The listing builds one solid part. Answer for the finished solid, in the listing's coordinates (mm). Coordinates: 2 decimals unless noted, no trailing zeros. Write each loop counter-clockwise with the first axis right and the second up, starting at its lowest first coordinate (ties: lowest second). Pieces come first, ordered by that corner, then holes.
(1) The part is cut by section B-B on x = 23. Determine the outline of the cut face in (y, z).
(2) The part is cut by section A-A on x = -36. Determine the outline of the cut face in (y, z), plus the area to 3 significant figures.
(3) Straight lines are drawn through the part: line 1 (X direction, y = -26.5, z = 0.5); line 2 (Y direction, x = 54, z = 0.8); line 3 (Y direction, x = 51.5, z = 2.55). For each, find the intervals that lie inside material, in ascending order.
(4) Given P1, Ø1.2, axis at y = 30, z = 3, coming from the -X side; P2, Ø2, axis at x = 57.5, z = 2.5, coming from the -Y side; P3, Ø2, axis at y = -22, z = 0.5, coming from the +X side, each flat-ended and moving along its own axis, determine where each tip first touches the part or whether it passes through.
(5) The part is cut by section C-C on z = 3.1. Give the number of separate pieces and of enclosed holes in the cut face, plus the area to 3 significant figures.
from build123d import *

# Parameters (mm, degrees)
EXTRUDE_1_DEPTH     = 4
CUT_EXTRUDE_1_DEPTH = 10


with BuildPart() as part:
    # 草图1 → 凸台-拉伸1 (new body)
    with BuildSketch(Plane.XY):
        Polygon((55.534285714, 24.23), (59.534285714, 24.23), (59.534285714, 16.23), (55.534285714, 16.23), (55.534285714, 6.73), (51.534285714, 6.73), (51.534285714, 8.08), (48.934285714, 8.08), (48.934285714, 6.73), (46.934285714, 6.73), (46.934285714, 3.73), (48.934285714, 3.73), (48.934285714, 2.38), (51.534285714, 2.38), (51.534285714, 3.73), (55.534285714, 3.73), (55.534285714, -5.77), (59.534285714, -5.77), (59.534285714, -13.77), (55.534285714, -13.77), (55.534285714, -23.27), (51.534285714, -23.27), (51.534285714, -21.92), (48.934285714, -21.92), (48.934285714, -23.27), (46.934285714, -23.27), (46.934285714, -26.27), (48.934285714, -26.27), (48.934285714, -27.62), (51.534285714, -27.62), (51.534285714, -26.27), (55.534285714, -26.27), (55.534285714, -35.77), (-70.465714286, -35.77), (-70.465714286, -26.27), (-66.465714286, -26.27), (-66.465714286, -27.62), (-63.865714286, -27.62), (-63.865714286, -26.27), (-61.865714286, -26.27), (-61.865714286, -23.27), (-63.865714286, -23.27), (-63.865714286, -21.92), (-66.465714286, -21.92), (-66.465714286, -23.27), (-70.465714286, -23.27), (-70.465714286, -13.77), (-74.465714286, -13.77), (-74.465714286, -5.77), (-70.465714286, -5.77), (-70.465714286, 3.73), (-66.465714286, 3.73), (-66.465714286, 2.38), (-63.865714286, 2.38), (-63.865714286, 3.73), (-61.865714286, 3.73), (-61.865714286, 6.73), (-63.865714286, 6.73), (-63.865714286, 8.08), (-66.465714286, 8.08), (-66.465714286, 6.73), (-70.465714286, 6.73), (-70.465714286, 16.23), (-74.465714286, 16.23), (-74.465714286, 24.23), (-70.465714286, 24.23), (-70.465714286, 33.73), (-66.465714286, 33.73), (-66.465714286, 32.38), (-63.865714286, 32.38), (-63.865714286, 33.73), (-61.865714286, 33.73), (-61.865714286, 36.73), (-63.865714286, 36.73), (-63.865714286, 38.08), (-66.465714286, 38.08), (-66.465714286, 36.73), (-70.465714286, 36.73), (-70.465714286, 46.23), (55.534285714, 46.23), (55.534285714, 36.73), (51.534285714, 36.73), (51.534285714, 38.08), (48.934285714, 38.08), (48.934285714, 36.73), (46.934285714, 36.73), (46.934285714, 33.73), (48.934285714, 33.73), (48.934285714, 32.38), (51.534285714, 32.38), (51.534285714, 33.73), (55.534285714, 33.73), align=None)
    extrude(amount=EXTRUDE_1_DEPTH)

    # 草图3 → 切除-拉伸1 (cut)
    with BuildSketch(Plane.XY.offset(4)):
        with BuildLine():
            Line((14.43310292, -15.539220042), (-51.863516332, 22.849447356))
            ThreePointArc((-51.863516332, 22.849447356), (-53.864614704, 22.851352584), (-54.865714286, 21.118667398))
            Line((-54.865714286, 21.118667398), (-54.865714286, -17.27))
            ThreePointArc((-54.865714286, -17.27), (-54.279927848, -18.684213562), (-52.865714286, -19.27))
            Line((-52.865714286, -19.27), (13.430904966, -19.27))
            ThreePointArc((13.430904966, -19.27), (15.362427671, -17.788864185), (14.43310292, -15.539220042))
        make_face()
        with BuildLine():
            Line((-28.362333538, 29.73), (37.934285714, 29.73))
            ThreePointArc((37.934285714, 29.73), (39.348499277, 29.144213562), (39.934285714, 27.73))
            Line((39.934285714, 27.73), (39.934285714, -10.658667398))
            ThreePointArc((39.934285714, -10.658667398), (38.933186133, -12.391352584), (36.932087761, -12.389447356))
            Line((36.932087761, -12.389447356), (-29.364531491, 25.999220042))
            ThreePointArc((-29.364531491, 25.999220042), (-30.293856242, 28.248864185), (-28.362333538, 29.73))
        make_face()
    extrude(amount=-CUT_EXTRUDE_1_DEPTH, mode=Mode.SUBTRACT)


solid = part.part
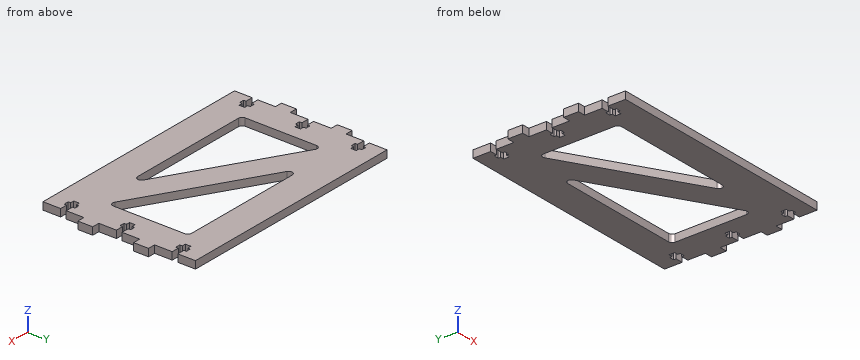
Model answer:
1. outline: (-35.77, 0) - (-4.32, 0) - (-4.32, 4) - (-35.77, 4) - close; (29.73, 0) - (46.23, 0) - (46.23, 4) - (29.73, 4) - close
2. outline: (-35.77, 0) - (-19.27, 0) - (-19.27, 4) - (-35.77, 4) - close; (13.66, 0) - (46.23, 0) - (46.23, 4) - (13.66, 4) - close
2. area: 196 mm2
3. line 1: x = -70.47 to -66.47, -63.87 to 48.93, 51.53 to 55.53
3. line 2: y = -35.77 to -26.27, -23.27 to 3.73, 6.73 to 33.73, 36.73 to 46.23
3. line 3: y = -35.77 to -27.62, -21.92 to 2.38, 8.08 to 32.38, 38.08 to 46.23
4. P1: stops at x = -70.47
4. P2: stops at y = -13.77
4. P3: stops at x = 55.53
5. separate pieces: 1
5. enclosed holes: 2
5. area: 6,970 mm2
